from build123d import *

# Parameters (mm, degrees)
SKETCH_1_R          = 40
EXTRUDE_1_DEPTH     = 40
SKETCH_2_R          = 26
EXTRUDE_2_DEPTH     = 3
SKETCH_3_R          = 29
EXTRUDE_3_DEPTH     = 3
FILLET_1_R          = 1
EXTRUDE_START       = 3
SKETCH_4_R          = 26
EXTRUDE_4_DEPTH     = 3
SKETCH_5_R          = 28
EXTRUDE_5_DEPTH     = 3
FILLET_2_R          = 1
SKETCH_6_W          = 20
SKETCH_6_H          = 30
FILLET_5_R          = 15
SKETCH_7_R          = 5.5
CUT_EXTRUDE_1_DEPTH = 77.837490849
SKETCH_8_R          = 2.4
CUT_EXTRUDE_2_DEPTH = 77.837490849


with BuildPart() as part:
    # 草图1 → 凸台-拉伸1 (new body)
    with BuildSketch(Plane(origin=(0, 0, 0), x_dir=(1, 0, 0), z_dir=(0, 1, 0))):
        with Locations(Location((0, 0, 0), (0, 0, 270))):
            Circle(SKETCH_1_R)
    extrude(amount=EXTRUDE_1_DEPTH)

    # 草图2 → 凸台-拉伸2 (add)
    with BuildSketch(Plane(origin=(0, 40, 0), x_dir=(1, 0, 0), z_dir=(0, 1, 0))):
        with Locations(Location((0, 0, 0), (0, 0, 270))):
            Circle(SKETCH_2_R)
    extrude(amount=EXTRUDE_2_DEPTH)

    # 草图3 → 凸台-拉伸3 (add)
    with BuildSketch(Plane(origin=(0, 43, 0), x_dir=(1, 0, 0), z_dir=(0, 1, 0))):
        with Locations(Location((0, 0, 0), (0, 0, 270))):
            Circle(SKETCH_3_R)
    extrude(amount=EXTRUDE_3_DEPTH)

    # 圆角1
    fillet_1_edges = [part.edges().sort_by_distance(p)[0] for p in [
        (0, 43, -26),
    ]]
    fillet(fillet_1_edges, radius=FILLET_1_R)

    # 草图4 → 凸台-拉伸4 (add)
    with BuildSketch(Plane.XZ.offset(EXTRUDE_START)):
        with Locations(Location((0, 0, 0), (0, 0, 90))):
            Circle(SKETCH_4_R)
    extrude(amount=-EXTRUDE_4_DEPTH)

    # 草图5 → 凸台-拉伸5 (add)
    with BuildSketch(Plane.XZ.offset(3)):
        with Locations(Location((0, 0, 0), (0, 0, 270))):
            Circle(SKETCH_5_R)
    extrude(amount=EXTRUDE_5_DEPTH)

    # 圆角2
    fillet_2_edges = [part.edges().sort_by_distance(p)[0] for p in [
        (0, -3, -26),
    ]]
    fillet(fillet_2_edges, radius=FILLET_2_R)

    # 草图6 → 切除-旋转1 (revolve, cut)
    with BuildSketch(Plane.XY, mode=Mode.PRIVATE) as cut_revolve_1_sk:
        with Locations((-30, 20)):
            Rectangle(SKETCH_6_W, SKETCH_6_H)
    revolve(cut_revolve_1_sk.sketch.rotate(Axis((0, -960, 0), (0, 1, 0)), 180), axis=Axis((0, -960, 0), (0, 1, 0)), mode=Mode.SUBTRACT)

    # 圆角5
    fillet_5_edges = [part.edges().sort_by_distance(p)[0] for p in [
        (-20, 5, 0),
        (-20, 35, 0),
    ]]
    fillet(fillet_5_edges, radius=FILLET_5_R - 0.0001)  # a hair under: the kernel refuses the full size

    # 草图7 → 切除-拉伸1 (cut, through all)
    with BuildSketch(Plane.XZ.offset(6)):
        with Locations(Location((0, 0, 0), (0, 0, 270))):
            Circle(SKETCH_7_R)
    extrude(amount=-CUT_EXTRUDE_1_DEPTH, mode=Mode.SUBTRACT)

    # 草图8 → 切除-拉伸2 (cut, through all)
    with BuildSketch(Plane.XZ.offset(6)):
        with Locations(Location((0, 12, 0), (0, 0, 270))):
            Circle(SKETCH_8_R)
        with Locations(Location((12, 0, 0), (0, 0, 270))):
            Circle(SKETCH_8_R)
        with Locations(Location((0, -12, 0), (0, 0, 270))):
            Circle(SKETCH_8_R)
        with Locations(Location((-12, 0, 0), (0, 0, 270))):
            Circle(SKETCH_8_R)
    extrude(amount=-CUT_EXTRUDE_2_DEPTH, mode=Mode.SUBTRACT)


solid = part.part
Design review of the part built by this model. Coordinates are the model's own, in mm. A direction names the side the tool comes from. Round coordinates to 2 decimals unless told otherwise and drop trailing zeros. Loops run counter-clockwise (first coordinate to the right, second up) from the corner with the lowest first, then second, coordinate; pieces in that order, holes last. Notation, with made-up numbers: (-17, 28.25) - (29, 28.25) arc R25 ccw to (29, 43.25) - close; hole circle Ø3 at (58.25, 73.25). An arc over 180 degrees is marked (long way). One line per question, with ' | ' between items.
1. For faces 1 (the face through (-0.2, 5, 35.4)), 2 (the face through (-11.107, 44.479, 26.789)), 3 (the face through (-27.334, -4.479, 6.07)), list the 3-axis set-ups (+Z, -Z, +X, -X, +Y, -Y) from which the entire face can be reached by the end or side of a thin tool; tool diameter is ignored.
Results are:
face 1: none | face 2: +Y | face 3: -Y
2. We need section B-B, the plane x = 0. State how many separate pieces and enclosed holes the cut face has, and give its area (3 significant figures).
Results are:
separate pieces: 4 | enclosed holes: 0 | area: 1,780 mm²
3. Draft analysis for pull direction X (two halves, no side actions). For faces 4 (the face through (0.106, 19.636, 14.398)), 5 (the face through (-9.62, 19.64, 0.31)), 6 (the face through (-15.821, 40.986, -20.633)), 7 (the face through (-26, 43, 8)), state which applies: released by +X, released by -X, zero draft, split by the parting line, or undercut.
Results are:
face 4: undercut | face 5: undercut | face 6: split by the parting line | face 7: zero draft
4. We need section A-A, the plane y = -1. State the section outline as (x, z) points.
Results are:
outline: circle Ø52 at (0, 0); hole circle Ø4.8 at (-12, 0); hole circle Ø11 at (0, 0); hole circle Ø4.8 at (0, -12); hole circle Ø4.8 at (0, 12); hole circle Ø4.8 at (12, 0)
5. We need section D-D, the plane y = 38. State the section outline as (x, z) points.
Results are:
outline: circle Ø80 at (0, 0); hole circle Ø4.8 at (-12, 0); hole circle Ø11 at (0, 0); hole circle Ø4.8 at (0, -12); hole circle Ø4.8 at (0, 12); hole circle Ø4.8 at (12, 0)
6. Clearance check with flat-ended pins moving along their axes: P1, Ø3, axis at x = 13.5, y = 9.5, coming from the -Z side; P2, Ø3, axis at y = 13.5, z = -17.5, coming from the +X side; P3, Ø12, axis at x = -21, y = 25.5, coming from the +Z side. State where each tip first meets the part, or that it passes through.
Results are:
P1: stops at z = -22.39 | P2: stops at x = 14.7 | P3: stops at z = 16.67
7. For L1, parallel to Z at x = -1.5, y = -1; L2, parallel to Y at x = 34.5, z = 7.5; L3, parallel to X at y = 1, z = -10, list the stretches that pass through material, from the lowest coordinate up. Write a range as [from, to].
Results are:
L1: z = [-25.96, -13.87], [-10.13, -5.29], [5.29, 10.13], [13.87, 25.96] | L2: y = [0, 5], [35, 40] | L3: x = [-38.73, -1.33], [1.33, 38.73]
